The drawing under review shows one solid part. Ordinate dimensions are in mm from its lowest x, y, z. Coordinates: 2 decimals unless noted, no trailing zeros. Order: outer loops, then holes, each group sorted by start corner. A loop starts at its lowest first (then second) coordinate and runs counter-clockwise, first axis right, second up.
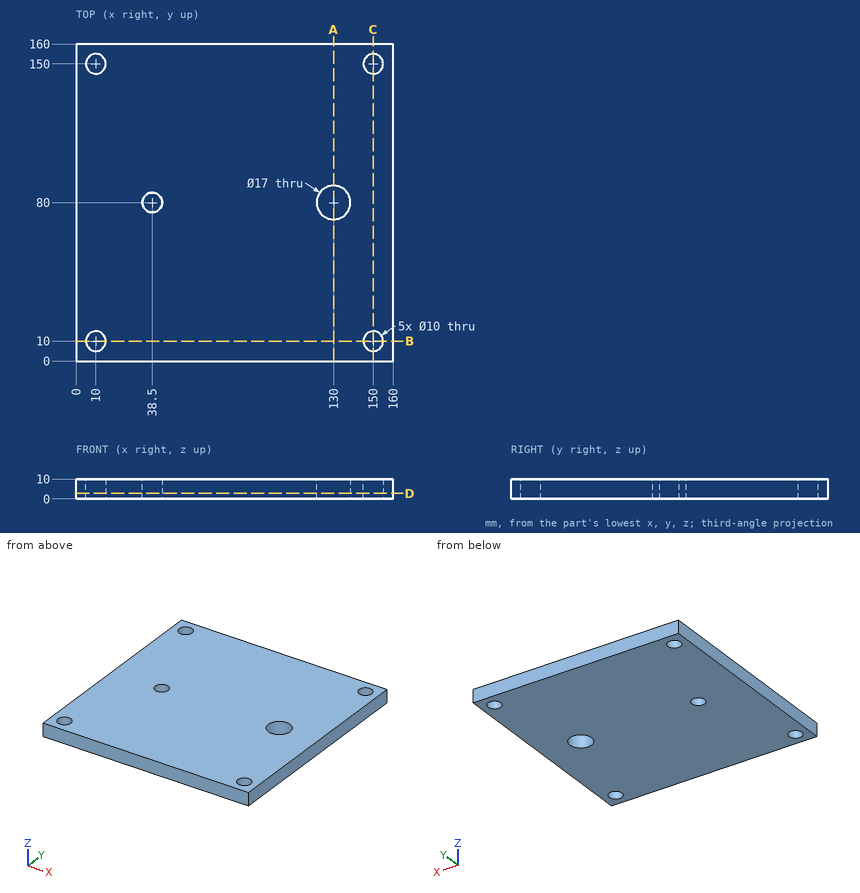
1. Insertion check: pin 1 (8 mm diameter, centred on x = 104.5, y = 39, fed in from -Z). The pin has a flat end and moves straight along its axis. Give the tip position at first contact, or say it passes through.
2. To check wall thickness, follow line 1 (X direction, y = 80.5, z = 1); line 2 (Y direction, x = 10, z = 6); line 3 (Y direction, x = 130, z = 3.5). State the ranges of each line that lie inside material, in increasing order.
3. Add section D-D (z = 2.75). Give the boundary of the cut face in (x, y), and give its area (3 significant figures).
4. Add section A-A (x = 130). Give the boundary of the cut face in (y, z).
5. Add section B-B (y = 10). Give the boundary of the cut face in (x, z).
Solution:
1. pin 1: stops at z = 0
2. line 1: x = 0 to 33.53, 43.47 to 121.51, 138.49 to 160
2. line 2: y = 0 to 5, 15 to 145, 155 to 160
2. line 3: y = 0 to 71.5, 88.5 to 160
3. outline: (0, 0) - (160, 0) - (160, 160) - (0, 160) - close; hole circle Ø10 at (10, 10); hole circle Ø10 at (10, 150); hole circle Ø10 at (38.5, 80); hole circle Ø17 at (130, 80); hole circle Ø10 at (150, 10); hole circle Ø10 at (150, 150)
3. area: 25,000 mm2
4. outline: (0, 0) - (71.5, 0) - (71.5, 10) - (0, 10) - close; (88.5, 0) - (160, 0) - (160, 10) - (88.5, 10) - close
5. outline: (0, 0) - (5, 0) - (5, 10) - (0, 10) - close; (15, 0) - (145, 0) - (145, 10) - (15, 10) - close; (155, 0) - (160, 0) - (160, 10) - (155, 10) - close
